Model file for the job. Use its own axes, mm. A direction names the side the tool comes from. Round coordinates to 2 decimals unless told otherwise and drop trailing zeros. Loops run counter-clockwise (first coordinate to the right, second up) from the corner with the lowest first, then second, coordinate; pieces in that order, holes last. Notation, with made-up numbers: (86.5, 15.5) - (91.5, 15.5) arc R9 ccw to (91.5, 22.5) - close; hole circle Ø3 at (19.25, 54). An arc over 180 degrees is marked (long way). Use one line per item in the form item = value.
from build123d import *

# Parameters (mm, degrees)
SKETCH1_W                                          = 93
SKETCH1_H                                          = 58
BOSS_EXTRUDE1_DEPTH                                = 42
SKETCH2_W                                          = 91
SKETCH2_H                                          = 54
CUT_EXTRUDE1_DEPTH                                 = 19
CUT_EXTRUDE2_DEPTH                                 = 18
SKETCH4_W                                          = 58
SKETCH4_H                                          = 42
BOSS_EXTRUDE2_DEPTH                                = 2
SKETCH5_W                                          = 34
SKETCH5_H                                          = 5
BOSS_EXTRUDE3_DEPTH                                = 15
CUT_EXTRUDE3_REACH                                 = 97
SKETCH6_W                                          = 13.999999973
SKETCH6_H                                          = 12.999999419
CUT_EXTRUDE4_DEPTH                                 = 18
CUT_EXTRUDE5_REACH                                 = 97
SKETCH8_W                                          = 16
SKETCH8_H                                          = 4
SKETCH9_W                                          = 22.000000328
SKETCH9_H                                          = 6
CUT_EXTRUDE6_DEPTH                                 = 74
SKETCH10_W                                         = 34
SKETCH10_H                                         = 5
BOSS_EXTRUDE4_DEPTH                                = 15
F_3_0_3_DIAMETER_HOLE1_D                           = 3
F_3_0_3_DIAMETER_HOLE1_DEPTH                       = 5
F_6_0_6_DIAMETER_HOLE1_D                           = 6
F_6_0_6_DIAMETER_HOLE1_DEPTH                       = 5
F_7_0_7_DIAMETER_HOLE1_D                           = 7
F_7_0_7_DIAMETER_HOLE1_DEPTH                       = 2
F_8_0_8_DIAMETER_HOLE1_D                           = 8
F_8_0_8_DIAMETER_HOLE1_DEPTH                       = 2
CBORE_FOR_M2_5_HEX_HEAD_MACHINE_SCREW1_D           = 3
CBORE_FOR_M2_5_HEX_HEAD_MACHINE_SCREW1_DEPTH       = 42
CBORE_FOR_M2_5_HEX_HEAD_MACHINE_SCREW1_CBORE_D     = 6
CBORE_FOR_M2_5_HEX_HEAD_MACHINE_SCREW1_CBORE_DEPTH = 3
FILLET1_R                                          = 2
FILLET2_R                                          = 6


with BuildPart() as part:
    # Sketch1 → Boss-Extrude1 (new body)
    with BuildSketch(Plane.XZ):
        with Locations((-1, 0)):
            Rectangle(SKETCH1_W, SKETCH1_H)
    extrude(amount=-BOSS_EXTRUDE1_DEPTH)

    # Sketch2 → Cut-Extrude1 (cut)
    with BuildSketch(Plane(origin=(0, 42, 0), x_dir=(-1, 0, 0), z_dir=(0, 1, 0))):
        Rectangle(SKETCH2_W, SKETCH2_H)
    extrude(amount=-CUT_EXTRUDE1_DEPTH, mode=Mode.SUBTRACT)

    # Sketch3 → Cut-Extrude2 (cut)
    with BuildSketch(Plane(origin=(0, 23, 0), x_dir=(-1, 0, 0), z_dir=(0, 1, 0))):
        Polygon((-35.5, -29), (-16.5, -29), (-16.5, -27), (45.5, -27), (45.5, 27), (-45.5, 27), (-45.5, -27), (-35.5, -27), align=None)
    extrude(amount=-CUT_EXTRUDE2_DEPTH, mode=Mode.SUBTRACT)

    # Sketch4 → Boss-Extrude2 (add)
    with BuildSketch(Plane(origin=(45.5, 0, 0), x_dir=(0, 0, -1), z_dir=(1, 0, 0))):
        with Locations((0, 21)):
            Rectangle(SKETCH4_W, SKETCH4_H)
    extrude(amount=BOSS_EXTRUDE2_DEPTH)

    # Sketch5 → Boss-Extrude3 (add)
    with BuildSketch(Plane(origin=(0, 0, -29), x_dir=(-1, 0, 0), z_dir=(0, 0, -1))):
        with Locations((0, 2.5)):
            Rectangle(SKETCH5_W, SKETCH5_H)
    extrude(amount=BOSS_EXTRUDE3_DEPTH)

    # Sketch6 → Cut-Extrude3 (cut, up to next)
    with BuildSketch(Plane.ZY.offset(47.5), mode=Mode.PRIVATE) as cut_extrude3_sk1:
        with Locations((-10.000000013, 35.50000029)):
            Rectangle(SKETCH6_W, SKETCH6_H)
    cut_extrude3_tool1 = extrude(cut_extrude3_sk1.sketch, amount=-CUT_EXTRUDE3_REACH, mode=Mode.PRIVATE) & part.part
    add(cut_extrude3_tool1.solids().sort_by_distance((-47.5, 35.5, -10))[0], mode=Mode.SUBTRACT)

    # Sketch7 → Cut-Extrude4 (cut, through all)
    with BuildSketch(Plane.XY.offset(-27)):
        Polygon((14.000000071, 10), (14.000000071, 24), (-37.500000057, 24), (-37.500000057, 15), (-23.000000328, 15), (-23.000000328, 10), align=None)
    extrude(amount=-CUT_EXTRUDE4_DEPTH, mode=Mode.SUBTRACT)

    # Sketch8 → Cut-Extrude5 (cut, up to next)
    with BuildSketch(Plane.ZY.offset(47.5), mode=Mode.PRIVATE) as cut_extrude5_sk1:
        with Locations((-8, 19)):
            Rectangle(SKETCH8_W, SKETCH8_H)
    cut_extrude5_tool1 = extrude(cut_extrude5_sk1.sketch, amount=-CUT_EXTRUDE5_REACH, mode=Mode.PRIVATE) & part.part
    add(cut_extrude5_tool1.solids().sort_by_distance((-47.5, 19, -8))[0], mode=Mode.SUBTRACT)

    # Sketch9 → Cut-Extrude6 (cut, through all)
    with BuildSketch(Plane.XY.offset(29)):
        with Locations((2.999999836, 17)):
            Rectangle(SKETCH9_W, SKETCH9_H)
    extrude(amount=-CUT_EXTRUDE6_DEPTH, mode=Mode.SUBTRACT)

    # Sketch10 → Boss-Extrude4 (add)
    with BuildSketch(Plane.XY.offset(29)):
        with Locations((0, 2.5)):
            Rectangle(SKETCH10_W, SKETCH10_H)
    extrude(amount=BOSS_EXTRUDE4_DEPTH)

    # Ø3.0 (3) Diameter Hole1
    with Locations(Plane(origin=(0, 5, 0), x_dir=(1, 0, 0), z_dir=(0, 1, 0))):
        with Locations((11, -38), (-11, 38), (-11, -38), (11, 38), (0, 22.5), (0, -22.5), (-39.5, -12.925), (-39.5, -9.425)):
            Hole(F_3_0_3_DIAMETER_HOLE1_D / 2, depth=F_3_0_3_DIAMETER_HOLE1_DEPTH)

    # Ø6.0 (6) Diameter Hole1
    with Locations(Plane(origin=(0, 5, 0), x_dir=(1, 0, 0), z_dir=(0, 1, 0))):
        with Locations((31.540291459, -20.22658296), (-31.540291459, -20.22658296), (31.540291459, 20.22658296), (-31.540291459, 20.22658296)):
            Hole(F_6_0_6_DIAMETER_HOLE1_D / 2, depth=F_6_0_6_DIAMETER_HOLE1_DEPTH)

    # Ø7.0 (7) Diameter Hole1
    with Locations(Plane.XY.offset(29)):
        with Locations((-18.000000328, 12), (-33.000000328, 12)):
            Hole(F_7_0_7_DIAMETER_HOLE1_D / 2, depth=F_7_0_7_DIAMETER_HOLE1_DEPTH)

    # Ø8.0 (8) Diameter Hole1
    with Locations(Plane.ZY.offset(47.5)):
        with Locations((11.228, 17.5)):
            Hole(F_8_0_8_DIAMETER_HOLE1_D / 2, depth=F_8_0_8_DIAMETER_HOLE1_DEPTH)

    # CBORE for M2.5 Hex Head Machine Screw1
    with Locations(Plane(origin=(0, 0, 0), x_dir=(-1, 0, 0), z_dir=(0, -1, 0))):
        with Locations((-39.5, -21), (39.5, -21), (-39.5, 21), (39.5, 21)):
            CounterBoreHole(CBORE_FOR_M2_5_HEX_HEAD_MACHINE_SCREW1_D / 2, CBORE_FOR_M2_5_HEX_HEAD_MACHINE_SCREW1_CBORE_D / 2, CBORE_FOR_M2_5_HEX_HEAD_MACHINE_SCREW1_CBORE_DEPTH, depth=CBORE_FOR_M2_5_HEX_HEAD_MACHINE_SCREW1_DEPTH)

    # Fillet1
    fillet1_edges = [part.edges().sort_by_distance(p)[0] for p in [
        (40.5, 5, -27),
        (45.5, 23.5, -27),
        (-45.5, 23.5, -27),
        (-14.5, 5, -27),
        (45.5, 5, 0),
        (45.5, 23.5, 27),
        (-45.5, 5, 0),
        (0, 5, 27),
        (-45.5, 23.5, 27),
        (17, 2.5, 29),
        (0, 5, 29),
        (-17, 2.5, 29),
        (47.5, 21, 29),
        (-0.25, 5, -29),
        (-17, 2.5, -29),
        (-47.5, 21, 29),
        (17, 2.5, -29),
        (47.5, 21, -29),
        (-47.5, 21, -29),
    ]]
    fillet(fillet1_edges, radius=FILLET1_R)

    # Fillet2
    fillet2_edges = [part.edges().sort_by_distance(p)[0] for p in [
        (-17, 2.5, 44),
        (17, 2.5, 44),
        (-17, 2.5, -44),
        (17, 2.5, -44),
    ]]
    fillet(fillet2_edges, radius=FILLET2_R)


solid = part.part
1. Cut at B-B, the plane x = 21. Give the cut face in (y, z).
Geometry check:
outline = (0, -29) - (5, -29) - (5, 25) arc R2 cw to (7, 27) - (42, 27) - (42, 29) - (0, 29) - close; (23, -29) - (42, -29) - (42, -27) - (23, -27) - close
2. Pull direction X, two halves, no side cores. Call faces 4 (the cylindrical face through (-46.486, 20.873, 9.078)), 5 (the flat face through (-17, 2, 34)), 6 (the flat face through (-45.5, 25, 0)): +X half, -X half, draft (parallel to the pull), parting line (faces both ways), or undercut.
Geometry check:
face_4 = draft
face_5 = -X half
face_6 = undercut
3. Cut at C-C, the plane x = -39.5. Give the number of separate pieces and of enclosed holes in the cut face, plus the area to 3 significant figures.
Geometry check:
separate_pieces = 5
enclosed_holes = 0
area = 362 mm^2
4. Wall check: probe 1 along Z at (x, y) = (-11, 1.05); probe 2 along X at (y, z) = (25, -1); probe 3 along Z at (x, y) = (39.5, 3.7). Give the ranges that are in metal, low to high.
Geometry check:
probe_1 = -44 to -39.5, -36.5 to 36.5, 39.5 to 44
probe_2 = -47.5 to -45.5, 45.5 to 47.5
probe_3 = -29 to -22.5, -19.5 to 19.5, 22.5 to 29
5. Tool access for faces 1 (the flat face through (-17, 2, -34)), 2 (the flat face through (17, 2, -34)), 3 (the flat face through (45.5, 25, 0)): list every direction of +Z, -Z, +X, -X, +Y, -Y with a clear straight run to the whole face (end or side of a thin tool).
Geometry check:
face_1 = -Z, -X, +Y, -Y
face_2 = -Z, +X, +Y, -Y
face_3 = +Y
6. Cut at D-D, the plane y = 32. Give the cut face in (x, z).
Geometry check:
outline = (-47.5, -27) arc R2 ccw to (-45.5, -29) - (45.5, -29) arc R2 ccw to (47.5, -27) - (47.5, 27) arc R2 ccw to (45.5, 29) - (-45.5, 29) arc R2 ccw to (-47.5, 27) - (-47.5, -3) - (-45.5, -3) - (-45.5, 25) arc R2 cw to (-43.5, 27) - (43.5, 27) arc R2 cw to (45.5, 25) - (45.5, -25) arc R2 cw to (43.5, -27) - (-43.5, -27) arc R2 cw to (-45.5, -25) - (-45.5, -17) - (-47.5, -17) - close
7. Flat gauge pins, fed straight in: pin 1 (4 mm diameter, centred on x = 11, z = -38, fed in from +Y); pin 2 (4 mm diameter, centred on x = -6, y = 32.5, fed in from +Z); pin 3 (2.5 mm diameter, centred on x = -39.5, z = 12.925, fed in from -Y); pin 4 (1 mm diameter, centred on y = 14.5, z = -28, fed in from -X). Where does each tip first touch, or does it go through?
Geometry check:
pin_1 = 5
pin_2 = 29
pin_3 = through
pin_4 = -47.44
8. Cut at A-A, the plane x = -6. Give the cut face in (y, z), plus the area to 3 significant figures.
Geometry check:
outline = (0, -44) - (5, -44) - (5, -31) arc R2 cw to (7, -29) - (10, -29) - (10, -27) - (7, -27) arc R2 cw to (5, -25) - (5, 25) arc R2 cw to (7, 27) - (14, 27) - (14, 29) - (7, 29) arc R2 cw to (5, 31) - (5, 44) - (0, 44) - close; (20, 27) - (42, 27) - (42, 29) - (20, 29) - close; (24, -29) - (42, -29) - (42, -27) - (24, -27) - close
area = 551 mm^2
